Geometry check sheet. Reference: the model listing, model coordinates, mm. Give positions to 0.01 mm unless a question says otherwise; leave off trailing zeros. Write each loop counter-clockwise with the first axis right and the second up, starting at its lowest first coordinate (ties: lowest second). Pieces come first, ordered by that corner, then holes. Notation, with made-up numbers: (87.5, 25.25) -> (117.5, 25.25) arc R5 cw to (117.5, 31.25) -> close; hole circle Ø7 at (15, 44). An arc over 180 degrees is marked (long way). Use a Markdown table: item, result. Add a question column.
from build123d import *

# Parameters (mm, degrees)
TOP_SKETCH_W             = 88
TOP_SKETCH_H             = 8
THICKNESS_EXTRUDE_DEPTH  = 0.1
PIN_HOLE_SKETCH_R        = 0.75
FIRST_PIN_HOLE_CUT_DEPTH = 89.362944722
PIN_HOLE_PATTERN_COUNT   = 23
PIN_HOLE_PATTERN_PITCH   = 4
POCKET_CUT_OUT_DEPTH     = 89.362944722
POCKET_DEPTH             = 88


with BuildPart() as part:
    # Top Sketch → Thickness Extrude (new body)
    with BuildSketch(Plane.XY):
        with Locations((-44, -4)):
            Rectangle(TOP_SKETCH_W, TOP_SKETCH_H)
    extrude(amount=-THICKNESS_EXTRUDE_DEPTH)

    # Pin Hole Sketch → First Pin Hole Cut (cut, through all)
    with BuildSketch(Plane.XY):
        with Locations((0, -1.75)):
            Circle(PIN_HOLE_SKETCH_R)
    first_pin_hole_cut = extrude(amount=-FIRST_PIN_HOLE_CUT_DEPTH, mode=Mode.SUBTRACT)

    # Pin Hole Pattern: First Pin Hole Cut ×23
    with Locations(*[(-i * PIN_HOLE_PATTERN_PITCH, 0, 0) for i in range(1, PIN_HOLE_PATTERN_COUNT)]):
        add(first_pin_hole_cut, mode=Mode.SUBTRACT)

    # Pocket Cut Out Sketch → Pocket Cut Out (cut, through all)
    with BuildSketch(Plane(origin=(0, 0, 0), x_dir=(0, 0, -1), z_dir=(1, 0, 0))):
        Polygon((0, -3.145020754), (0, -7.354979246), (2.4, -6.481450684), (2.4, -4.018549316), align=None)
    extrude(amount=-POCKET_CUT_OUT_DEPTH, mode=Mode.SUBTRACT)


with BuildPart() as pocket_cut_out_piece_1:
    # of the separate pieces the step leaves, piece 1, a body of its own (pocket_cut_out_pieces)
    add(part.part.solids().sort_by_distance((-88, 0, 0))[0])



with BuildPart() as pocket_cut_out_piece_2:
    # of the separate pieces the step leaves, piece 2, a body of its own (pocket_cut_out_pieces)
    add(part.part.solids().sort_by_distance((0, -7.354979246, 0))[0])


with BuildPart() as pocket_cut_out_piece_1_1:
    add(pocket_cut_out_piece_1.part)

    add(pocket_cut_out_piece_2.part)  # Pocket merges Pocket Cut Out piece 2
    # Pocket Sketch → Pocket (add, through all)
    with BuildSketch(Plane(origin=(0, 0, 0), x_dir=(0, 0, -1), z_dir=(1, 0, 0))):
        Polygon((0, -3.145020754), (2.4, -4.018549316), (2.4, -6.481450684), (0, -7.354979246), (0.1, -7.425), (2.5, -6.551471438), (2.5, -3.948528562), (0.1, -3.075), align=None)
    extrude(amount=-POCKET_DEPTH)


solid = pocket_cut_out_piece_1_1.part
1) Sectioned sample at B-B, the plane z = -1.8. Enter the section's corners in (x, y).
2) Gauge pin test, flat ends, axial feed: P1, Ø1.5, axis at x = -32.5, y = -3, coming from the +Z side; P2, Ø1.7, axis at x = -32, y = -1.75, coming from the -Z side; P3, Ø1.4, axis at x = -76, y = -1.75, coming from the -Z side; P4, Ø1, axis at x = -75.5, y = -5, coming from the +Z side. Record the tip position at first contact, or that the pin passes through.
3) Sectioned sample at A-A, the plane x = -40. Enter the section's corners in (y, z) (3 decimals), and give its area (3 significant figures).
4) Sectioned sample at C-C, the plane x = -74.5. Enter the section's corners in (y, z) (3 decimals), and give its area (3 significant figures).
Check values:
| question | item | result |
|---|---|---|
| 1 | outline | (-88, -6.81) -> (0, -6.81) -> (0, -6.7) -> (-88, -6.7) -> close; (-88, -3.8) -> (0, -3.8) -> (0, -3.69) -> (-88, -3.69) -> close |
| 2 | P1 | z = 0 |
| 2 | P2 | z = -0.1 |
| 2 | P3 | through |
| 2 | P4 | z = -2.4 |
| 3 | outline | (-8, -0.1) -> (-7.425, -0.1) -> (-6.551, -2.5) -> (-3.949, -2.5) -> (-3.075, -0.1) -> (-2.5, -0.1) -> (-2.5, 0) -> (-3.145, 0) -> (-4.019, -2.4) -> (-6.481, -2.4) -> (-7.355, 0) -> (-8, 0) -> close; (-1, -0.1) -> (0, -0.1) -> (0, 0) -> (-1, 0) -> close |
| 3 | area | 0.986 mm² |
| 4 | outline | (-8, -0.1) -> (-7.425, -0.1) -> (-6.551, -2.5) -> (-3.949, -2.5) -> (-3.075, -0.1) -> (0, -0.1) -> (0, 0) -> (-3.145, 0) -> (-4.019, -2.4) -> (-6.481, -2.4) -> (-7.355, 0) -> (-8, 0) -> close |
| 4 | area | 1.14 mm² |
